```python
from build123d import *

# Parameters (mm, degrees)
BOSS_EXTRUDE1_DEPTH = 4
SKETCH2_R           = 1.5
CUT_EXTRUDE1_DEPTH  = 4
CUT_EXTRUDE5_DEPTH  = 34
CUT_EXTRUDE6_DEPTH  = 34
SKETCH6_R           = 1.5
CUT_EXTRUDE7_DEPTH  = 10


with BuildPart() as part:
    # Sketch1 → Boss-Extrude1 (new body)
    with BuildSketch(Plane.XY):
        Polygon((0, 0), (-40, 0), (-40, 24.5), (-13, 24.5), (-13, 49), (100, 49), (100, 0), align=None)
    extrude(amount=BOSS_EXTRUDE1_DEPTH)

    # Sketch2 → Cut-Extrude1 (cut)
    with BuildSketch(Plane.XY.offset(4)):
        with Locations((39.857429038, 36.5)):
            Circle(SKETCH2_R)
        with Locations((69.057429038, 27)):
            Circle(SKETCH2_R)
        with Locations((69.057429038, 46)):
            Circle(SKETCH2_R)
    extrude(amount=-CUT_EXTRUDE1_DEPTH, mode=Mode.SUBTRACT)

    # Sketch4 → Cut-Extrude5 (cut)
    with BuildSketch(Plane(origin=(0, 0, -4), x_dir=(-1, 0, 0), z_dir=(0, 0, -1))):
        Polygon((-80.710769515, 31.7), (-79.671539031, 33.5), (-80.710769515, 35.3), (-82.789230485, 35.3), (-83.828460969, 33.5), (-82.789230485, 31.7), align=None)
        Polygon((-47.210769515, 31.7), (-46.171539031, 33.5), (-47.210769515, 35.3), (-49.289230485, 35.3), (-50.328460969, 33.5), (-49.289230485, 31.7), align=None)
        Polygon((-47.210769515, 13.7), (-46.171539031, 15.5), (-47.210769515, 17.3), (-49.289230485, 17.3), (-50.328460969, 15.5), (-49.289230485, 13.7), align=None)
        Polygon((-80.710769515, 13.7), (-79.671539031, 15.5), (-80.710769515, 17.3), (-82.789230485, 17.3), (-83.828460969, 15.5), (-82.789230485, 13.7), align=None)
    extrude(amount=-CUT_EXTRUDE5_DEPTH, mode=Mode.SUBTRACT)

    # Sketch5 → Cut-Extrude6 (cut)
    with BuildSketch(Plane(origin=(0, 0, 0), x_dir=(-1, 0, 0), z_dir=(0, 0, -1))):
        Polygon((4.7511107, 37.15), (6.2522214, 39.75), (4.7511107, 42.35), (1.7488893, 42.35), (0.2477786, 39.75), (1.7488893, 37.15), align=None)
        Polygon((-25.7488893, 37.15), (-24.2477786, 39.75), (-25.7488893, 42.35), (-28.7511107, 42.35), (-30.2522214, 39.75), (-28.7511107, 37.15), align=None)
        Polygon((-25.7488893, 6.65), (-24.2477786, 9.25), (-25.7488893, 11.85), (-28.7511107, 11.85), (-30.2522214, 9.25), (-28.7511107, 6.65), align=None)
        Polygon((4.7511107, 6.65), (6.2522214, 9.25), (4.7511107, 11.85), (1.7488893, 11.85), (0.2477786, 9.25), (1.7488893, 6.65), align=None)
    extrude(amount=-CUT_EXTRUDE6_DEPTH, mode=Mode.SUBTRACT)

    # Sketch6 → Cut-Extrude7 (cut)
    with BuildSketch(Plane.XY.offset(4)):
        with Locations((-33, 12)):
            Circle(SKETCH6_R)
        with Locations((93, 12)):
            Circle(SKETCH6_R)
    extrude(amount=-CUT_EXTRUDE7_DEPTH, mode=Mode.SUBTRACT)


solid = part.part
```
Read the model definition and answer for the solid it produces. Units are mm, in the model's axes. A direction names the side the tool comes from. Round coordinates to 2 decimals unless told otherwise and drop trailing zeros. Write each loop counter-clockwise with the first axis right and the second up, starting at its lowest first coordinate (ties: lowest second). Pieces come first, ordered by that corner, then holes. Notation, with made-up numbers: (-15, 11) -> (-2, 11) arc R22 cw to (-2, 38) -> close; hole circle Ø11 at (49.5, 39.5). An arc over 180 degrees is marked (long way). Answer in a Markdown table with one row per item. Add a question column.
1) Which of the six approach directions +Z, -Z, +X, -X, +Y, -Y give full straight-line access (tool end or side, diameter ignored) to faces 5 (the face through (-0.988, 7.968, 1.972)), 6 (the face through (100, 25, 2))?
2) Determine the mould class of faces 1 (the face through (-40, 12, 2)), 2 (the face through (29, 0, 2)), 3 (the face through (69.864, 28.265, 2.028)), 4 (the face through (-3, 37.15, 2)) for opening direction X: pulls with the +X half, pulls with the -X half, needs draft (parallel to the pull), parting line crosses it, or undercut.
3) Find section C-C, the plane z = 2.4. State how many separate pieces and enclosed holes the cut face has, and give its area (3 significant figures).
4) Consider line 1 (X direction, y = 9, z = 1.7); line 2 (Y direction, x = 93, z = 3.15); line 3 (X direction, y = 34.5, z = 2.45). Determine where each line is inside the solid, lowest interval first.
5) Find section B-B, the plane x = 93. Determine the outline of the cut face in (y, z), and give its area (3 significant figures).
6) Find section A-A, the plane x = -33. Determine the outline of the cut face in (y, z).
7) Given P1, Ø2.5, axis at x = -33, y = 12, coming from the +Z side, flat-ended and moving along its own axis, determine where the tip first touches the part or whether it passes through.
Findings below:
| question | item | result |
|---|---|---|
| 1 | face 5 | +Z, -Z |
| 1 | face 6 | +Z, -Z, +X, +Y, -Y |
| 2 | face 1 | pulls with the -X half |
| 2 | face 2 | needs draft |
| 2 | face 3 | undercut |
| 2 | face 4 | undercut |
| 3 | separate pieces | 1 |
| 3 | enclosed holes | 13 |
| 3 | area | 6,020 mm² |
| 4 | line 1 | -40 to -6.11, -0.39 to 24.39, 30.11 to 100 |
| 4 | line 2 | 0 to 10.5, 13.5 to 49 |
| 4 | line 3 | -13 to 46.75, 49.75 to 80.25, 83.25 to 100 |
| 5 | outline | (0, 0) -> (10.5, 0) -> (10.5, 4) -> (0, 4) -> close; (13.5, 0) -> (49, 0) -> (49, 4) -> (13.5, 4) -> close |
| 5 | area | 184 mm² |
| 6 | outline | (0, 0) -> (10.5, 0) -> (10.5, 4) -> (0, 4) -> close; (13.5, 0) -> (24.5, 0) -> (24.5, 4) -> (13.5, 4) -> close |
| 7 | P1 | through |
